from build123d import *

# Parameters (mm, degrees)
SKETCH_1_W          = 1200
SKETCH_1_H          = 2445
EXTRUDE_1_DEPTH     = 12.5
SKETCH_3_W          = 400
SKETCH_3_H          = 802.75
CUT_EXTRUDE_2_DEPTH = 2724.63383185


with BuildPart() as part:
    # Эскиз1 → Бобышка-Вытянуть1 (new body)
    with BuildSketch(Plane.XY):
        with Locations((-600, 1222.5)):
            Rectangle(SKETCH_1_W, SKETCH_1_H)
    extrude(amount=-EXTRUDE_1_DEPTH)

    # Эскиз3 → Вырез-Вытянуть2 (cut, through all)
    with BuildSketch(Plane.XY):
        with Locations((-1000, 1301.375)):
            Rectangle(SKETCH_3_W, SKETCH_3_H)
    extrude(amount=-CUT_EXTRUDE_2_DEPTH, mode=Mode.SUBTRACT)


solid = part.part
Work out the finished part from the listing and answer in its coordinate system (mm). Give positions to 0.01 mm unless a question says otherwise; leave off trailing zeros. Order: outer loops, then holes, each group sorted by start corner. A loop starts at its lowest first (then second) coordinate and runs counter-clockwise, first axis right, second up. Notation, with made-up numbers: (30, -33) -> (85, -33) arc R18 cw to (85, -26) -> close; hole circle Ø1 at (-27.5, -27). An arc over 180 degrees is marked (long way). Answer as a JSON object with one key per item and string values. Group by question number.
1. A flat-ended cylindrical pin translates along its axis: pin 1 Ø4 at (y, z) = (1074, -10) entering from -X. Find the tip coordinate at first contact, or state that the pin passes through.
2. Consider line 1 along X through (y, z) = (1144, -3.25). Determine where the line is inside the solid, lowest interval first. Write a range as [from, to].
3. Section C-C on y = 1545.5 is taken. Determine the outline of the cut face in (x, z).
4. Section A-A on x = -1021.5 is taken. Determine the outline of the cut face in (y, z).
5. Section B-B on z = -6 is taken. Determine the outline of the cut face in (x, y), plus the area to 3 significant figures.
Result sheet:
{
 "1": {"pin 1": "stops at x = -800"},
 "2": {"line 1": "x = [-800, 0]"},
 "3": {"outline": "(-800, -12.5) -> (0, -12.5) -> (0, 0) -> (-800, 0) -> close"},
 "4": {"outline": "(0, -12.5) -> (900, -12.5) -> (900, 0) -> (0, 0) -> close; (1702.75, -12.5) -> (2445, -12.5) -> (2445, 0) -> (1702.75, 0) -> close"},
 "5": {"outline": "(-1200, 0) -> (0, 0) -> (0, 2445) -> (-1200, 2445) -> (-1200, 1702.75) -> (-800, 1702.75) -> (-800, 900) -> (-1200, 900) -> close", "area": "2,610,000 mm^2"}
}
